Part model, mm, in its own coordinate system. Face numbers are marked on the shaded views. A direction names the side the tool comes from. Round coordinates to 2 decimals unless told otherwise and drop trailing zeros. Order: outer loops, then holes, each group sorted by start corner. A loop starts at its lowest first (then second) coordinate and runs counter-clockwise, first axis right, second up. Notation, with made-up numbers: M 29,12.5 L 65,12.5 A18 ccw 65,46.5 Z; hole C 89.25,59 d1. An arc over 180 degrees is marked long. Write each question's results on one line, items separated by ' | '. Start each with the question number.
1. Which spindle directions (+Z, -Z, +X, -X, +Y, -Y) get a long thin tool onto all of the face, cutting with end or side? Do the marked faces 1, 2 and 3. Say none if no direction does.
2. Band-saw the part on A-A, the plane y = 0. List the corners of the cut face in (x, z), then the cut area to 3 significant figures.
3. Probe L1, parallel to Z at x = 1.05, y = -0.4; L2, parallel to X at y = 0.1, z = 10.75; L3, parallel to X at y = -2.1, z = 13. List the from-to ranges inside material, lowest first. Write a range as [from, to].
4. Band-saw the part on C-C, the plane z = 14.5. List the corners of the cut face in (x, y).
5. Drop a flat-ended pin along its axis: pin 1 Ø1.5 at (y, z) = (1, 1.5) entering from +X. Give the stop position or say it passes through.
6. Band-saw the part on D-D, the plane z = -1. List the corners of the cut face in (x, y), then the cut area to 3 significant figures.
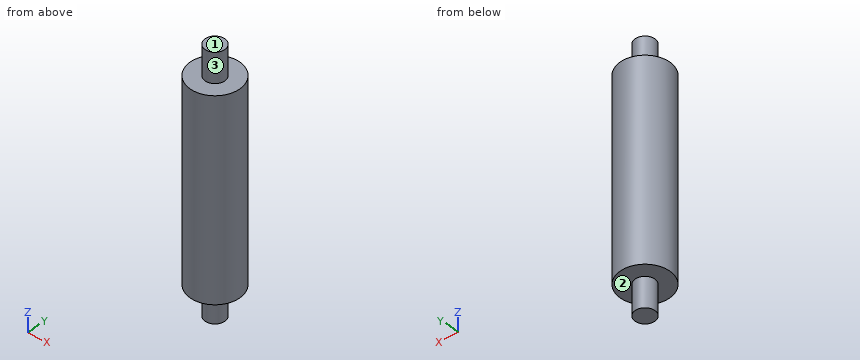
Autodesk Inventor part; units mm, degrees
ref_plane "YZ Plane" through (0, 0, 0) normal (1, 0, 0) x (0, 1, 0)
ref_plane "XZ Plane" through (0, 0, 0) normal (0, 1, 0) x (-1, 0, 0)
ref_plane "XY Plane" through (0, 0, 0) normal (0, 0, 1) x (1, 0, 0)
sketch "Sketch1" plane through (0, 0, 0) normal (0, 0, 1) x (1, 0, 0)
  circle A0 centre (0, 0) radius 2.5
  dimension "d0" = 5
extrude "Extrusion1" add sketch "Sketch1" along normal blind 20
sketch "Sketch2" plane through (0, 0, 20) normal (0, 0, 1) x (1, 0, 0)
  circle A0 centre (0, 0) radius 2.5
  circle A1 centre (0, 0) radius 1
  dimension "d3" = 2
extrude "Extrusion2" add sketch "Sketch2" along normal blind 3 contours A1
sketch "Sketch3" plane through (0, 0, 0) normal (0, 0, -1) x (-1, 0, 0)
  circle A0 centre (0, 0) radius 1
  dimension "d6" = 2
extrude "Extrusion3" add sketch "Sketch3" along normal blind 3
properties part number "Bone-2cm"
Solution:
1) face 1: +Z, +X, -X, +Y, -Y | face 2: -Z | face 3: +Z
2) outline: M -2.5,0 L -1,0 L -1,-3 L 1,-3 L 1,0 L 2.5,0 L 2.5,20 L 1,20 L 1,23 L -1,23 L -1,20 L -2.5,20 Z | area: 112 mm^2
3) L1: [0, 20] | L2: [-2.5, 2.5] | L3: [-1.36, 1.36]
4) outline: C 0,0 d5
5) pin 1: x = 2.49
6) outline: C 0,0 d2 | area: 3.14 mm^2
